The figure shows three views and two pictorial views of one solid part (mm, origin at its lowest corner). Answer the questions. A direction names the side the tool comes from. Coordinates: 2 decimals unless noted, no trailing zeros. Loops run counter-clockwise (first coordinate to the right, second up) from the corner with the lowest first, then second, coordinate; pieces in that order, holes last.
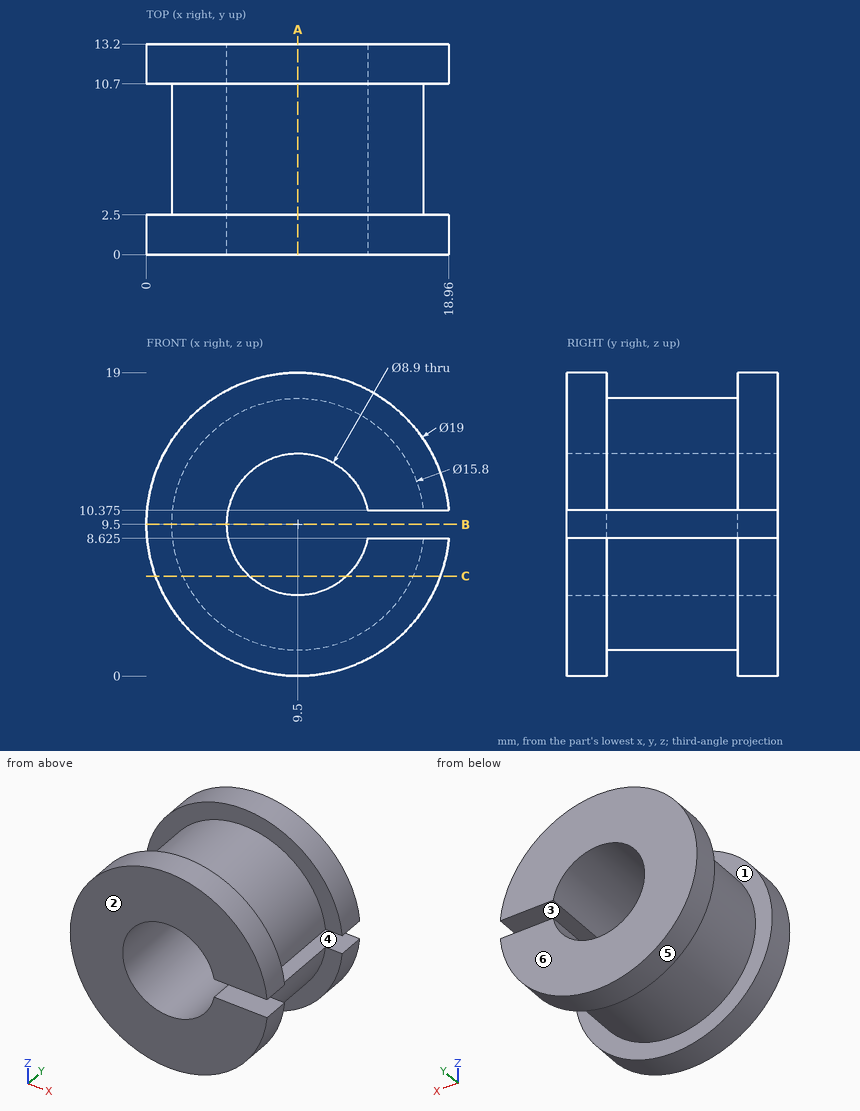
Q1. Which of the six approach directions +Z, -Z, +X, -X, +Y, -Y give full straight-line access (tool end or side, diameter ignored) to the marked faces 1, 2 and 3?
Findings below:
face 1: none
face 2: +Z, -Z, +X, -X, -Y
face 3: +X, +Y, -Y
Q2. Flat-ended cylindrical pins translate along their axes: pin 1 Ø6 at (y, z) = (3, 14) entering from +X; pin 2 Ø2 at (x, y) = (16, 4.5) entering from -Z; pin 3 Ø7 at (x, z) = (9.5, 9.5) entering from +Y; pin 4 Ø5.5 at (x, y) = (16, 3.5) entering from +Z (1 decimal). Find the tip coordinate at first contact, or state that the pin passes through.
Findings below:
pin 1: stops at x = 18.87
pin 2: stops at z = 3.83
pin 3: passes through
pin 4: stops at z = 18.1
Q3. Determine the mould class of the marked faces 4, 5 and 6 for opening direction Z: +Z half, -Z half, draft (parallel to the pull), parting line (faces both ways), or undercut.
Findings below:
face 4: undercut
face 5: parting line
face 6: draft
Q4. A cutting plane is placed at C-C (z = 6.25). Give the vertices of the cut face in (x, y), then the cut area to 3 significant figures.
Findings below:
outline: (0.57, 0) - (6.46, 0) - (6.46, 13.2) - (0.57, 13.2) - (0.57, 10.7) - (2.3, 10.7) - (2.3, 2.5) - (0.57, 2.5) - close; (12.54, 0) - (18.43, 0) - (18.43, 2.5) - (16.7, 2.5) - (16.7, 10.7) - (18.43, 10.7) - (18.43, 13.2) - (12.54, 13.2) - close
area: 127 mm2
Q5. A cutting plane is placed at B-B (z = 9.5). Give the vertices of the cut face in (x, y).
Findings below:
outline: (0, 0) - (5.05, 0) - (5.05, 13.2) - (0, 13.2) - (0, 10.7) - (1.6, 10.7) - (1.6, 2.5) - (0, 2.5) - close
Q6. A cutting plane is placed at A-A (x = 9.5). Give the vertices of the cut face in (y, z).
Findings below:
outline: (0, 0) - (2.5, 0) - (2.5, 1.6) - (10.7, 1.6) - (10.7, 0) - (13.2, 0) - (13.2, 5.05) - (0, 5.05) - close; (0, 13.95) - (13.2, 13.95) - (13.2, 19) - (10.7, 19) - (10.7, 17.4) - (2.5, 17.4) - (2.5, 19) - (0, 19) - close
Q7. Straight lines are drawn through the part: probe 1 along Z at (x, y) = (9.5, 7.5); probe 2 along Y at (x, z) = (3.75, 3.25); probe 3 along X at (y, z) = (4.5, 9.5). For each, find the intervals that lie inside material, in ascending order.
Findings below:
probe 1: z = 1.6 to 5.05, 13.95 to 17.4
probe 2: y = 0 to 2.5, 10.7 to 13.2
probe 3: x = 1.6 to 5.05
